from build123d import *

# Parameters (mm, degrees)
F2_R     = 1
F3_DEPTH = 6


with BuildPart() as f1:
    # F0 (on Front) → F1 (revolve)
    with BuildSketch(Plane.XZ):
        with BuildLine():
            Line((32.712799, 2), (-37.858998, 2))
            ThreePointArc((-37.858998, 2), (-42.358375, 3.863703), (-45.323099, 0))
            Line((-45.323099, 0), (40.176901, 0))
            ThreePointArc((40.176901, 0), (37.212177, 3.863703), (32.712799, 2))
        make_face()
    revolve(axis=Axis((-2.573099, 0, 0), (1, 0, 0)))

    # F2 (on Front) → F3 (join, symmetric)
    with BuildSketch(Plane.XZ):
        with Locations((-41.323099, 0)):
            Circle(F2_R)
        with Locations((36.176901, 0)):
            Circle(F2_R)
    extrude(amount=F3_DEPTH, both=True)


solid = f1.part
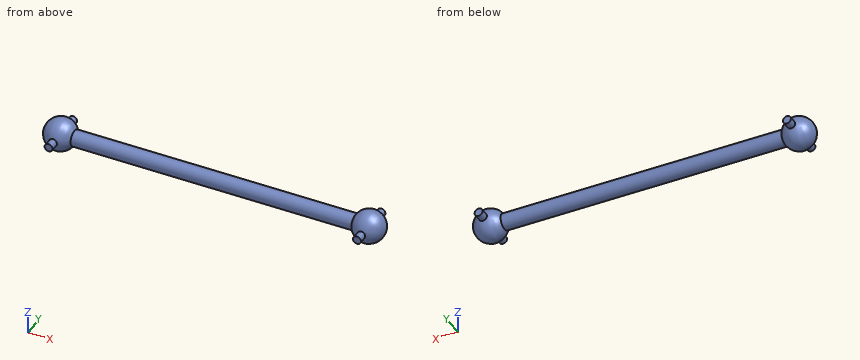
The model under review builds one solid part; all positions refer to its coordinate system, in mm. Round coordinates to 2 decimals unless told otherwise and drop trailing zeros. Write each loop counter-clockwise with the first axis right and the second up, starting at its lowest first coordinate (ties: lowest second). Pieces come first, ordered by that corner, then holes. Notation, with made-up numbers: (50.25, 76.5) -> (67.25, 76.5) arc R9 ccw to (67.25, 91.5) -> close; hole circle Ø5 at (-11, 60.5). An arc over 180 degrees is marked (long way). Answer as a JSON object with one key per item and string values.
1. We need section B-B on x = 4. State the section outline as (y, z) points, and give its area (3 significant figures).
Results found:
{"outline": "circle Ø4 at (0, 0)", "area": "12.6 mm^2"}
2. To check wall thickness, follow line 1 along X through (y, z) = (-3, -1.5); line 2 along X through (y, z) = (2.25, -2.75); line 3 along Y through (x, z) = (16, 0.25). State the ranges of each line that lie inside material, in increasing order.
Results found:
{"line 1": "x = -43.5 to -39.14, 34 to 38.36", "line 2": "x = -43.16 to -39.49, 34.34 to 38.01", "line 3": "y = -1.98 to 1.98"}
3. We need section A-A on y = -5. State the section outline as (x, z) points.
Results found:
{"outline": "circle Ø2 at (-41.32, 0); circle Ø2 at (36.18, 0)"}
4. Clearance check with flat-ended pins moving along their axes: pin 1 (1 mm diameter, centred on x = -11, y = -2, fed in from +Z); pin 2 (2 mm diameter, centred on y = -4, z = 1.5, fed in from -X); pin 3 (4 mm diameter, centred on y = -2.5, z = 1, fed in from -X). State where each tip first meets the part, or that it passes through.
Results found:
{"pin 1": "stops at z = 1.32", "pin 2": "stops at x = -43.62", "pin 3": "stops at x = -45.26"}
